from build123d import *

# Parameters (mm, degrees)
SKETCH1_W                 = 682.625
SKETCH1_H                 = 203.2
BASE_FLANGE1_DEPTH        = 3.175
EDGE_FLANGE1_DEPTH        = 682.625
EDGE_FLANGE3_DEPTH        = 669.925
EDGE_FLANGE3_BEND_DEPTH   = 179.941884035
EDGE_FLANGE3_BEND_2_DEPTH = 179.941884035
EDGE_FLANGE3_BEND_3_DEPTH = 147.556884035
EDGE_FLANGE3_BEND_4_DEPTH = 147.556884035
EDGE_FLANGE4_DEPTH        = 670.465


# Sheet-metal steps are written as plain solids
with BuildPart() as part:
    # Sketch1 → Base-Flange1 (new body)
    with BuildSketch(Plane.XY):
        Rectangle(SKETCH1_W, SKETCH1_H)
    extrude(amount=-BASE_FLANGE1_DEPTH)

    # Edge-Flange1 section (across the edge) → Edge-Flange1 (add)
    with BuildSketch(Plane(origin=(341.3125, -102.87, -3.175), x_dir=(0, 0.6872977622647618, -0.7263757884083493), z_dir=(-1, 0, 0))):
        with BuildLine():
            Line((-3.175, 0.398115965), (-3.175, 151.13))
            Line((-3.175, 151.13), (0, 151.13))
            Line((0, 151.13), (0, 0.398115965))
            ThreePointArc((0, 0.398115965), (0.070920943, 0.02823476), (0.273624212, -0.289181798))
            Line((0.273624212, -0.289181798), (0.872868158, -0.922497251))
            Line((0.872868158, -0.922497251), (-1.43337497, -3.104667646))
            Line((-1.43337497, -3.104667646), (-2.032618917, -2.471352193))
            ThreePointArc((-2.032618917, -2.471352193), (-2.878905063, -1.146138066), (-3.175, 0.398115965))
        make_face()
    extrude(amount=EDGE_FLANGE1_DEPTH)

    # Edge-Flange3 section (across the edge) → Edge-Flange3 (add)
    with BuildSketch(Plane(origin=(-334.9625, 102.87, -3.175), x_dir=(0, -1, 0), z_dir=(1, 0, 0))):
        with BuildLine():
            Line((-3.175, 1), (-3.175, 17.78))
            Line((-3.175, 17.78), (0, 17.78))
            Line((0, 17.78), (0, 1))
            ThreePointArc((0, 1), (0.292893219, 0.292893219), (1, 0))
            Line((1, 0), (1.27, 0))
            Line((1.27, 0), (1.27, -3.175))
            Line((1.27, -3.175), (1, -3.175))
            ThreePointArc((1, -3.175), (-1.952170811, -1.952170811), (-3.175, 1))
        make_face()
    extrude(amount=EDGE_FLANGE3_DEPTH)

    # Edge-Flange3 section 2 (across the edge) → Edge-Flange3 bend (add)
    with BuildSketch(Plane(origin=(-342.5825, -84.691884035, -3.175), x_dir=(1, 0, 0), z_dir=(0, 1, 0))):
        with BuildLine():
            Line((-3.175, 1), (-3.175, 17.78))
            Line((-3.175, 17.78), (0, 17.78))
            Line((0, 17.78), (0, 1))
            ThreePointArc((0, 1), (0.292893219, 0.292893219), (1, 0))
            Line((1, 0), (1.27, 0))
            Line((1.27, 0), (1.27, -3.175))
            Line((1.27, -3.175), (1, -3.175))
            ThreePointArc((1, -3.175), (-1.952170811, -1.952170811), (-3.175, 1))
        make_face()
    extrude(amount=EDGE_FLANGE3_BEND_DEPTH)

    # Edge-Flange3 section 3 (across the edge) → Edge-Flange3 bend 2 (add)
    with BuildSketch(Plane(origin=(342.5825, 95.25, -3.175), x_dir=(-1, 0, 0), z_dir=(0, -1, 0))):
        with BuildLine():
            Line((-3.175, 1), (-3.175, 17.78))
            Line((-3.175, 17.78), (0, 17.78))
            Line((0, 17.78), (0, 1))
            ThreePointArc((0, 1), (0.292893219, 0.292893219), (1, 0))
            Line((1, 0), (1.27, 0))
            Line((1.27, 0), (1.27, -3.175))
            Line((1.27, -3.175), (1, -3.175))
            ThreePointArc((1, -3.175), (-1.952170811, -1.952170811), (-3.175, 1))
        make_face()
    extrude(amount=EDGE_FLANGE3_BEND_2_DEPTH)

    # Edge-Flange3 section 4 (across the edge) → Edge-Flange3 bend 3 (add)
    with BuildSketch(Plane(origin=(-342.5825, -212.647172902, -107.046310811), x_dir=(1, 0, 0), z_dir=(1.4731097295439079e-15, 0.7263757884083494, 0.6872977622647618))):
        with BuildLine():
            Line((-3.175, 1), (-3.175, 17.78))
            Line((-3.175, 17.78), (0, 17.78))
            Line((0, 17.78), (0, 1))
            ThreePointArc((0, 1), (0.292893219, 0.292893219), (1, 0))
            Line((1, 0), (1.27, 0))
            Line((1.27, 0), (1.27, -3.175))
            Line((1.27, -3.175), (1, -3.175))
            ThreePointArc((1, -3.175), (-1.952170811, -1.952170811), (-3.175, 1))
        make_face()
    extrude(amount=EDGE_FLANGE3_BEND_3_DEPTH)

    # Edge-Flange3 section 5 (across the edge) → Edge-Flange3 bend 4 (add)
    with BuildSketch(Plane(origin=(342.5825, -105.465424926, -5.630794607), x_dir=(-1, 0, 0), z_dir=(-1.4731097295439075e-15, -0.7263757884083494, -0.6872977622647617))):
        with BuildLine():
            Line((-3.175, 1), (-3.175, 17.78))
            Line((-3.175, 17.78), (0, 17.78))
            Line((0, 17.78), (0, 1))
            ThreePointArc((0, 1), (0.292893219, 0.292893219), (1, 0))
            Line((1, 0), (1.27, 0))
            Line((1.27, 0), (1.27, -3.175))
            Line((1.27, -3.175), (1, -3.175))
            ThreePointArc((1, -3.175), (-1.952170811, -1.952170811), (-3.175, 1))
        make_face()
    extrude(amount=EDGE_FLANGE3_BEND_4_DEPTH)

    # Edge-Flange4 section (across the edge) → Edge-Flange4 (add)
    with BuildSketch(Plane(origin=(335.2325, -213.569670153, -107.919178969), x_dir=(0, 0.9999999999999994, 3.7524568563540583e-08), z_dir=(-1, 0, 0))):
        with BuildLine():
            Line((-3.175, 0.430496527), (-3.175, 17.78))
            Line((-3.175, 17.78), (0, 17.78))
            Line((0, 17.78), (0, 0.430496527))
            ThreePointArc((0, 0.430496527), (0.081496398, 0.035083916), (0.312702265, -0.295879288))
            Line((0.312702265, -0.295879288), (0.922497284, -0.872868123))
            Line((0.922497284, -0.872868123), (-1.259673025, -3.179111334))
            Line((-1.259673025, -3.179111334), (-1.869468044, -2.602122498))
            ThreePointArc((-1.869468044, -2.602122498), (-2.83475254, -1.220351122), (-3.175, 0.430496527))
        make_face()
    extrude(amount=EDGE_FLANGE4_DEPTH)


solid = part.part
Can you work these out from the model? Positions are in its coordinate system, mm. A direction names the side the tool comes from. Coordinates: 2 decimals unless noted, no trailing zeros. Order: outer loops, then holes, each group sorted by start corner. A loop starts at its lowest first (then second) coordinate and runs counter-clockwise, first axis right, second up. Notation, with made-up numbers: M 11.5,89.5 L 46.5,89.5 A21 ccw 46.5,96.5 Z; hole C -22.5,-27 d7. An arc over 180 degrees is marked long. Answer as CSV lines item,"result".
(1) If we mould it in two halves opening along Y, with no side actions, what happens to faces 1 (the cylindrical face through (344.502, -159.67, -54.187)), 2 (the flat face through (-343.998, -100.346, -11.042)), 3 (the flat face through (343.998, -100.346, -11.042)), 4 (the cylindrical face through (-342.3, -159.6, -57.27))? For each: released by +Y, released by -Y, zero draft, split by the parting line, or undercut.
Geometry check:
face 1,"released by -Y"
face 2,"undercut"
face 3,"undercut"
face 4,"released by +Y"
(2) On a 3-axis mill with a long thin cutter (end or side, diameter ignored), from which of +Z, -Z, +X, -X, +Y, -Y can I reach the whole of each face in a straight line? I mean faces 5 (the flat face through (-342.582, -153, -64)), 6 (the flat face through (-5, 102.87, -13)), 7 (the flat face through (5, -213.57, -117)). Say none if no direction works.
Geometry check:
face 5,"-Z, +Y"
face 6,"-Z, +X, -X"
face 7,"-Z, +X, -X, +Y"
(3) Suppose I cut it at A-A on x = 84. Please give me the cut outline in (y, z) (3 decimals), plus the area to 3 significant figures.
Geometry check:
outline,"M -216.745,-125.699 L -213.57,-125.699 L -213.57,-108.35 A1 cw -213.257,-107.623 L -103.159,-3.449 A1 cw -102.472,-3.175 L 101.87,-3.175 A1 cw 102.87,-4.175 L 102.87,-20.955 L 106.045,-20.955 L 106.045,-4.175 A4.175 ccw 101.87,0 L -102.472,0 A4.175 ccw -105.341,-1.142 L -215.439,-105.317 A4.175 ccw -216.745,-108.35 Z"
area,"1,260 mm^2"
(4) I'm going to push flat-ended pins straight in: pin 1 (1 mm diameter, centred on x = 336.5, z = -1.5, fed in from +Y); pin 2 (6 mm diameter, centred on x = 101.5, y = -118, fed in from -Z); pin 3 (1 mm diameter, centred on x = -113, z = -73.5, fed in from -Y); pin 4 (10 mm diameter, centred on x = -25.5, y = 51, fed in from +Z). Where does each tip first touch, or does it pass through?
Geometry check:
pin 1,"y = 101.6"
pin 2,"z = -20.33"
pin 3,"y = -182.34"
pin 4,"z = 0"
(5) Please list where these lines run through material, in increasing order: L1, parallel to Z at x = -211, y = 50.5 (3 decimals); L2, parallel to Y at x = -142, z = -11 (3 decimals); L3, parallel to X at y = -167, z = -68.5.
Geometry check:
L1,"-3.175 to 0"
L2,"-115.759 to -111.14, 102.87 to 106.045"
L3,"-345.76 to -342.58, 342.58 to 345.76"
